Autodesk Inventor part; units mm, degrees
ref_plane "YZ Plane" through (0, 0, 0) normal (1, 0, 0) x (0, 1, 0)
ref_plane "XZ Plane" through (0, 0, 0) normal (0, 1, 0) x (-1, 0, 0)
ref_plane "XY Plane" through (0, 0, 0) normal (0, 0, 1) x (1, 0, 0)
ref_plane "작업 평면1" through (0, 0, -34) normal (0, 0, -1) x (-1, 0, 0)
sketch "스케치1" plane through (0, 0, -34) normal (0, 0, -1) x (-1, 0, 0)
  circle A0 centre (17.3, -18) radius 1.35
  line L0 (20.1, -44.6) -> (20.1, 8.5)
  line L1 (14.5, -42) -> (14.5, 11.5)
  circle A1 centre (17.3, 4) radius 1.35
  circle A2 centre (17.3, -18) radius 1.45
  circle A3 centre (17.3, 4) radius 1.45
  line L2 (14.7, -42) -> (14.7, 11.5)
  line L3 (14.7, 11.5) -> (20.1, 8.5)
  line L4 (14.7, -20.9546) -> (32.7, -20.9546)
  line L5 (32.7, -20.9546) -> (32.7, 8.5)
  line L6 (32.7, 8.5) -> (20.1, 8.5)
  line L7 (32.7, -20.9546) -> (26.7, -20.9546)
  line L8 (26.7, -20.9546) -> (26.7, 8.5)
  line L9 (26.7, 8.5) -> (32.7, 8.5)
  line L10 (32.7, 8.5) -> (32.7, -20.9546)
  line L11 (20.1, 8.5) -> (14.7, 8.5)
  point P0 (0, 0)
  dimension "d0" = 0.1
  dimension "d1" = 0.1
  dimension "d2" = 0.2
  dimension "d3" = 18
  dimension "d8" = 6
extrude "돌출1" add sketch "스케치1" along normal blind 3 contours L4 L2 L11 L0 | L0 L6 L8 L4 | L8 L6 L5 L4 | A2 | A3
sketch "스케치2" plane through (0, 0, -34) normal (0, 0, 1) x (1, 0, 0)
  line L0 (-20.1, 8.5) -> (-14.7, 11.5)
  line L1 (-14.7, 8.5) -> (-14.7, -20.9546)
  line L2 (-20.1, -44.6) -> (-20.1, 8.5)
  line L3 (-32.7, 8.5) -> (-14.7, 8.5)
  line L4 (-32.7, -20.9546) -> (-32.7, 8.5)
  line L5 (-14.7, -20.9546) -> (-32.7, -20.9546)
  line L6 (-20.1, -20.9546) -> (-32.7, -20.9546)
  line L7 (-32.7, -20.9546) -> (-32.7, 8.5)
  line L8 (-32.7, 8.5) -> (-20.1, 8.5)
  line L9 (-20.1, 8.5) -> (-20.1, -20.9546)
  line L10 (-20.1, -20.9546) -> (-14.7, -20.9546)
  line L11 (-14.7, 11.5) -> (-20.1, 8.5)
  circle A0 centre (-17.3, -18) radius 1.45
  circle A1 centre (-17.3, 4) radius 1.35
  circle A2 centre (-17.3, 4) radius 1.45
  circle A3 centre (-17.3, 4) radius 1.45
  circle A4 centre (-17.3, -18) radius 1.45
  point P0 (0, 0)
ref_plane "작업 평면2" through (0, 0, 0) normal (0, 0, 1) x (1, 0, 0)
sketch "스케치3" plane through (0, 0, 0) normal (0, 0, 1) x (1, 0, 0)
  line L0 (-32.7, 8.5) -> (-14.7, 8.5)
  line L1 (-32.7, -20.9546) -> (-32.7, 8.5)
  line L2 (-14.7, -20.9546) -> (-32.7, -20.9546)
  line L3 (-14.7, 8.5) -> (-14.7, -20.9546)
  line L4 (-20.1, -20.9546) -> (-32.7, -20.9546)
  line L5 (-32.7, -20.9546) -> (-32.7, 8.5)
  line L6 (-32.7, 8.5) -> (-20.1, 8.5)
  line L7 (-20.1, 8.5) -> (-20.1, -20.9546)
  line L8 (-32.7, -20.9546) -> (-20.1, -20.9546)
  line L9 (-20.1, -20.9546) -> (-20.1, 8.5)
  line L10 (-20.1, 8.5) -> (-32.7, 8.5)
  line L11 (-32.7, 8.5) -> (-32.7, -20.9546)
  line L12 (-20.1, -20.9546) -> (-14.7, -20.9546)
  line L13 (-14.7, 8.5) -> (-14.7, -20.9546)
  line L14 (-14.7, 11.5) -> (-20.1, 8.5)
  circle A0 centre (-17.3, -18) radius 1.45
  circle A1 centre (-17.3, 4) radius 1.45
  circle A2 centre (-17.3, 4) radius 1.35
  circle A3 centre (-17.3, 4) radius 1.35
  circle A4 centre (-17.3, -18) radius 1.35
  point P0 (0, 0)
  dimension "d25" = 2.7
  dimension "d26" = 2.7
extrude "돌출2" add sketch "스케치3" along normal blind 3 contours L0 L7 L2 L1 | L0 L3 L2 L7 | A0 | A1
sketch "스케치4" plane through (0, 0, -34) normal (0, 0, 1) x (1, 0, 0)
  line L0 (-14.7, -20.9546) -> (-14.7, 8.5)
  line L1 (-14.7, 8.5) -> (-32.7, 8.5)
  line L2 (-32.7, 8.5) -> (-32.7, -20.9546)
  line L3 (-32.7, -20.9546) -> (-14.7, -20.9546)
  line L4 (-32.7, 8.5) -> (-26.7, 8.5)
  line L5 (-26.7, -20.9546) -> (-32.7, -20.9546)
  line L6 (-32.7, -20.9546) -> (-32.7, 8.5)
  line L7 (-32.7, 8.5) -> (-29.7, 8.5)
  line L8 (-29.7, 8.5) -> (-29.7, -20.9546)
  line L9 (-29.7, -20.9546) -> (-32.7, -20.9546)
  line L10 (-32.7, -20.9546) -> (-32.7, 8.5)
  point P0 (0, 0)
  point P1 (-29.7, -20.9546)
  dimension "d9" = 6
  dimension "d23" = 3
extrude "돌출3" add sketch "스케치4" along normal up to surface (34 mm away) contours L3 L2 L1 L8
sketch "스케치6" plane through (-32.7, -20.9546, -37) normal (-1, 0, 0) x (0, 0, 1)
  line L0 (40, 29.4546) -> (0, 29.4546)
  line L1 (0, 0) -> (0, 29.4546)
  line L2 (0, 0) -> (40, 0)
  line L3 (40, 29.4546) -> (40, 0)
  circle A0 centre (20, 14.7273) radius 1.6
  point P0 (37, 20.9546)
  dimension "d24" = 3.2
extrude "돌출5" cut sketch "스케치6" against normal blind 10 contours A0
fillet "모깎기1" radius 1 4 edges at (-32.7, -6.2273, 3) (-32.7, -6.2273, -37) (-29.7, -6.2273, -34) (-29.7, -6.2273, 0)
properties part number "3D_ankle1" material "PMMA 플라스틱"
Work out the finished part from the listing and answer in its coordinate system (mm). A direction names the side the tool comes from. Round coordinates to 2 decimals unless told otherwise and drop trailing zeros. Loops run counter-clockwise (first coordinate to the right, second up) from the corner with the lowest first, then second, coordinate; pieces in that order, holes last. Notation, with made-up numbers: (-10.75, 26.5) - (9.25, 26.5) arc R30 ccw to (9.25, 48.5) - close; hole circle Ø8 at (3, -5). An arc over 180 degrees is marked (long way). Use one line per item in the form item = value. Start each with the question number.
(1) Find section A-A on x = -17.3. Determine the outline of the cut face in (y, z), and give its area (3 significant figures).
(2) Determine the mould class of faces 3 (the face through (-29.415, -6.433, -33.699)), 4 (the face through (-16.053, -17.483, 1.479)), 5 (the face through (-30, 8.5, -19)) for opening direction Y: +Y half, -Y half, draft (parallel to the pull), parting line (faces both ways), or undercut.
(3) Flat-ended cylindrical pins translate along their axes: P1, Ø2, axis at x = -17.3, y = -18, coming from the +Z side; P2, Ø6, axis at y = 2, z = -27, coming from the +X side. Find the tip coordinate at first contact, or state that the pin passes through.
(4) Find section B-B on x = -20.5. Determine the outline of the cut face in (y, z).
(5) Find section D-D on y = 4. Determine the outline of the cut face in (x, z).
(6) Which of the six approach directions +Z, -Z, +X, -X, +Y, -Y give full straight-line access (tool end or side, diameter ignored) to faces 1 (the face through (-32.399, -6.021, -36.715)), 2 (the face through (-29.7, -9, -17))?
(7) Consider line 1 (Y direction, x = -17.3, z = -36.35); line 2 (Z direction, x = -24.25, y = -15.75); line 3 (X direction, y = -8.75, z = -21). Determine where each line is inside the solid, lowest interval first.
(8) Find section C-C on z = -17. Determine the outline of the cut face in (x, y).
Answer list:
q1.outline = (-20.95, -37) - (-19.35, -37) - (-19.35, -34) - (-20.95, -34) - close; (-20.95, 0) - (-19.35, 0) - (-19.35, 3) - (-20.95, 3) - close; (-16.65, -37) - (2.65, -37) - (2.65, -34) - (-16.65, -34) - close; (-16.65, 0) - (2.65, 0) - (2.65, 3) - (-16.65, 3) - close; (5.35, -37) - (8.5, -37) - (8.5, -34) - (5.35, -34) - close; (5.35, 0) - (8.5, 0) - (8.5, 3) - (5.35, 3) - close
q1.area = 144 mm^2
q2.face_3 = draft
q2.face_4 = undercut
q2.face_5 = +Y half
q3.P1 = through
q3.P2 = -29.7
q4.outline = (-20.95, -37) - (8.5, -37) - (8.5, -34) - (-20.95, -34) - close; (-20.95, 0) - (8.5, 0) - (8.5, 3) - (-20.95, 3) - close
q5.outline = (-32.7, -36) arc R1 ccw to (-31.7, -37) - (-18.65, -37) - (-18.65, -34) - (-28.7, -34) arc R1 cw to (-29.7, -33) - (-29.7, -1) arc R1 cw to (-28.7, 0) - (-18.65, 0) - (-18.65, 3) - (-31.7, 3) arc R1 ccw to (-32.7, 2) - close; (-15.95, -37) - (-14.7, -37) - (-14.7, -34) - (-15.95, -34) - close; (-15.95, 0) - (-14.7, 0) - (-14.7, 3) - (-15.95, 3) - close
q6.face_1 = -Z, -X, +Y, -Y
q6.face_2 = +X, +Y, -Y
q7.line_1 = -20.95 to -19.35, -16.65 to 2.65, 5.35 to 8.5
q7.line_2 = -37 to -34, 0 to 3
q7.line_3 = -32.7 to -29.7
q8.outline = (-32.7, -20.95) - (-29.7, -20.95) - (-29.7, -7.83) - (-32.7, -7.83) - close; (-32.7, -4.63) - (-29.7, -4.63) - (-29.7, 8.5) - (-32.7, 8.5) - close
